```python
from build123d import *

# Parameters (mm, degrees)
SKETCH_1_R      = 1.9
EXTRUDE_1_DEPTH = 13
SKETCH_2_W      = 13.159242617
SKETCH_2_H      = 30
EXTRUDE_2_DEPTH = 10


with BuildPart() as part:
    # 草图1 → 凸台-拉伸1 (new body)
    with BuildSketch(Plane(origin=(0, 0, 0), x_dir=(1, 0, 0), z_dir=(0, 1, 0))):
        Polygon((-23.5, -5.5), (-23.5, -21.5), (23.5, -21.5), (23.5, -5.5), (23.5, 5.5), (-23.5, 5.5), align=None)
        with Locations(Location((20.159242617, 2.75, 0), (0, 0, 90))):
            Circle(SKETCH_1_R, mode=Mode.SUBTRACT)
        with Locations(Location((-8.840757383, 2.75, 0), (0, 0, 90))):
            Circle(SKETCH_1_R, mode=Mode.SUBTRACT)
        with Locations(Location((-19.340757383, 2.75, 0), (0, 0, 90))):
            Circle(SKETCH_1_R, mode=Mode.SUBTRACT)
        with Locations(Location((0, -2.75, 0), (0, 0, 90))):
            Circle(SKETCH_1_R, mode=Mode.SUBTRACT)
        with Locations(Location((12, -2.75, 0), (0, 0, 90))):
            Circle(SKETCH_1_R, mode=Mode.SUBTRACT)
    extrude(amount=EXTRUDE_1_DEPTH)

    # 草图2 → 凸台-拉伸2 (add)
    with BuildSketch(Plane.XY.offset(21.5)):
        with Locations((-16.920378692, -15)):
            Rectangle(SKETCH_2_W, SKETCH_2_H)
    extrude(amount=-EXTRUDE_2_DEPTH)


solid = part.part
```
For this review, take the finished solid that the model builds, in its own axes (mm). Coordinates: 2 decimals unless noted, no trailing zeros. Order: outer loops, then holes, each group sorted by start corner. A loop starts at its lowest first (then second) coordinate and runs counter-clockwise, first axis right, second up. Notation, with made-up numbers: (-6, -39) -> (41, -39) arc R11 ccw to (41, -22) -> close; hole circle Ø10 at (84.5, 38). An arc over 180 degrees is marked (long way). Use CSV: the item, a comma, the result in double quotes. Start each with the question number.
Item 1: We need section D-D, the plane x = -13. Give the boundary of the cut face in (y, z).
Item 2: Insertion check: pin 1 (6 mm diameter, centred on x = 0, z = 2.75, fed in from -Y); pin 2 (4.5 mm diameter, centred on x = 20.16, z = -2.75, fed in from +Y); pin 3 (3 mm diameter, centred on y = -16.5, z = 14, fed in from +X); pin 4 (10.5 mm diameter, centred on x = -19, y = -8, fed in from -Z). Each pin has a flat end and moves straight along its axis. Give the tip position at first contact, or say it passes through.
Item 3: Draft analysis for pull direction X (two halves, no side actions). For faces 1 (the face through (-10.341, -15, 17)), 2 (the face through (-17, -15, 11.5)), 3 (the face through (18.275, 6.409, -2.503)), state which applies: pulls with the +X half, pulls with the -X half, needs draft (parallel to the pull), parting line crosses it, or undercut.
Item 4: We need section C-C, the plane z = 2.75. Give the boundary of the cut face in (x, y), then the cut area to 3 significant figures.
Item 5: We need section A-A, the plane z = -2.75. Give the boundary of the cut face in (x, y).
Item 6: Wall thickness on probe 1 along X at (y, z) = (8, -2.75); probe 2 along X at (y, z) = (8.25, 2.75); probe 3 along Z at (x, y) = (-18.5, -7): over which ranges is each line inside the solid? List them lowest first.
Item 7: We need section B-B, the plane x = 12. Give the boundary of the cut face in (y, z).
Derived:
1,outline,"(-30, 11.5) -> (0, 11.5) -> (0, -5.5) -> (13, -5.5) -> (13, 21.5) -> (-30, 21.5) -> close"
2,pin 1,"stops at y = 0"
2,pin 2,"stops at y = 13"
2,pin 3,"stops at x = -10.34"
2,pin 4,"stops at z = 11.5"
3,face 1,"pulls with the +X half"
3,face 2,"needs draft"
3,face 3,"undercut"
4,outline,"(-23.5, 0) -> (-1.9, 0) -> (-1.9, 13) -> (-23.5, 13) -> close; (1.9, 0) -> (10.1, 0) -> (10.1, 13) -> (1.9, 13) -> close; (13.9, 0) -> (23.5, 0) -> (23.5, 13) -> (13.9, 13) -> close"
4,area,"512 mm^2"
5,outline,"(-23.5, 0) -> (-21.24, 0) -> (-21.24, 13) -> (-23.5, 13) -> close; (-17.44, 0) -> (-10.74, 0) -> (-10.74, 13) -> (-17.44, 13) -> close; (-6.94, 0) -> (18.26, 0) -> (18.26, 13) -> (-6.94, 13) -> close; (22.06, 0) -> (23.5, 0) -> (23.5, 13) -> (22.06, 13) -> close"
6,probe 1,"x = -23.5 to -21.24, -17.44 to -10.74, -6.94 to 18.26, 22.06 to 23.5"
6,probe 2,"x = -23.5 to -1.9, 1.9 to 10.1, 13.9 to 23.5"
6,probe 3,"z = 11.5 to 21.5"
7,outline,"(0, -5.5) -> (13, -5.5) -> (13, 0.85) -> (0, 0.85) -> close; (0, 4.65) -> (13, 4.65) -> (13, 21.5) -> (0, 21.5) -> close"
